Read the model definition and answer for the solid it produces. Units are mm, in the model's axes. Face numbers are marked on the shaded views. Coordinates: 2 decimals unless noted, no trailing zeros. Loops run counter-clockwise (first coordinate to the right, second up) from the corner with the lowest first, then second, coordinate; pieces in that order, holes last. Notation, with made-up numbers: M 47,54 L 95,54 A19 cw 95,73 Z; hole C 55,36.5 d8. An arc over 180 degrees is marked long. One line per item, written item: value. Start each with the question number.
1. The part is cut by section A-A (y = 53). Write down the section's boundary in (x, z), then the cut area to 3 significant figures.
2. The part is cut by section B-B (x = 76). Write down the section's boundary in (y, z), then the cut area to 3 significant figures.
3. Flat-ended cylindrical pins translate along their axes: pin 1 (4.5 mm diameter, centred on x = 32.21, y = 39.51, fed in from +Z); pin 2 (2 mm diameter, centred on y = 47.5, z = 3, fed in from -X); pin 3 (1 mm diameter, centred on x = 90.5, z = 3, fed in from +Y); pin 4 (1.1 mm diameter, centred on y = 164.5, z = 3.5, fed in from +X). Find the tip coordinate at first contact, or state that the pin passes through.
4. Consider probe 1 along Y at (x, z) = (40.5, 0.5); probe 2 along Y at (x, z) = (33.5, 1.75); probe 3 along X at (y, z) = (42, 4.5). Determine where each line is inside the solid, lowest interval first.
5. Determine the mould class of the marked faces 1 and 2 for opening direction Z: +Z half, -Z half, draft (parallel to the pull), parting line (faces both ways), or undercut.
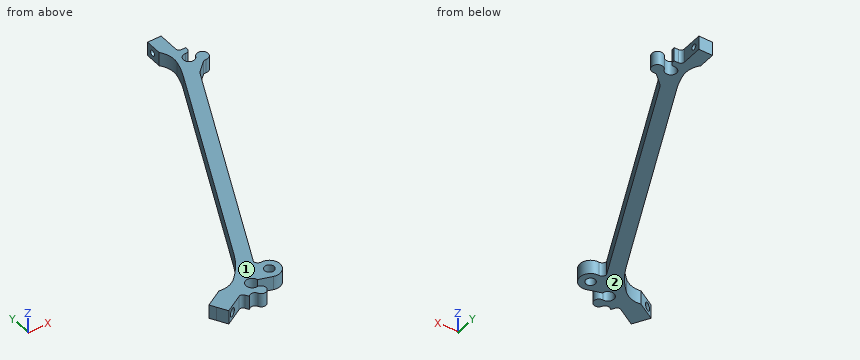
```python
from build123d import *

# Parameters (mm, degrees)
SKETCH1_R                 = 2.159
BOSS_EXTRUDE1_DEPTH       = 6.35
SKETCH2_R                 = 1.8288
CUT_EXTRUDE1_DEPTH        = 192.647335654
SKETCH3_R                 = 0.635
CUT_EXTRUDE2_DEPTH        = 192.476049021
FILLET1_R                 = 1.5875
FILLET2_R                 = 38.1
M3X0_5_TAPPED_HOLE1_D     = 2.5
M3X0_5_TAPPED_HOLE1_DEPTH = 7.50062
M3X0_5_TAPPED_HOLE1_TIP   = 0.751075774
CORTAR_EXTRUIR1_DEPTH     = 10
CROQUIS8_W                = 8.969129367
CROQUIS8_H                = 6.35
CROQUIS8_R                = 1.8288
SALIENTE_EXTRUIR3_DEPTH   = 3
CROQUIS7_W                = 6.35
CROQUIS7_H                = 7.383174339
CROQUIS7_R                = 1.25
SALIENTE_EXTRUIR4_DEPTH   = 3
REDONDEO1_R               = 10


with BuildPart() as part:
    # Sketch1 → Boss-Extrude1 (new body)
    with BuildSketch(Plane.XY):
        with BuildLine():
            Line((15.834722261, 31.434493723), (25.183466494, 36.831993723))
            Line((25.183466494, 36.831993723), (26.929716494, 33.8074))
            Line((26.929716494, 33.8074), (27.78608986, 34.301827393))
            ThreePointArc((27.78608986, 34.301827393), (29.23868298, 34.44834582), (30.311273673, 33.457869357))
            ThreePointArc((30.311273673, 33.457869357), (34.825897025, 33.143744407), (32.428977808, 36.9824))
            ThreePointArc((32.428977808, 36.9824), (30.032058591, 40.821055593), (34.546681944, 40.506930643))
            ThreePointArc((34.546681944, 40.506930643), (34.984344673, 39.889437479), (35.639187691, 39.509928464))
            Line((35.639187691, 39.509928464), (40.774282272, 37.860721969))
            ThreePointArc((40.774282272, 37.860721969), (47.368100791, 42.064756802), (42.017768622, 47.767939879))
            ThreePointArc((42.017768622, 47.767939879), (40.437125748, 48.5456558), (40.301653082, 50.302050149))
            Line((40.301653082, 50.302050149), (87.227692295, 149.642175178))
            ThreePointArc((87.227692295, 149.642175178), (87.739785188, 150.497310852), (88.408996906, 151.235993347))
            Line((88.408996906, 151.235993347), (92.404798917, 154.858512458))
            ThreePointArc((92.404798917, 154.858512458), (93.060884875, 155.23586864), (93.814481006, 155.3061491))
            ThreePointArc((93.814481006, 155.3061491), (96.343832869, 159.058865136), (91.821, 158.9024))
            ThreePointArc((91.821, 158.9024), (87.298167131, 158.745934864), (89.827518994, 162.4986509))
            ThreePointArc((89.827518994, 162.4986509), (91.22159212, 162.932303457), (91.821, 164.263545213))
            Line((91.821, 164.263545213), (91.821, 165.2524))
            Line((91.821, 165.2524), (88.3285, 165.2524))
            Line((88.3285, 165.2524), (88.3285, 176.0474))
            Line((88.3285, 176.0474), (85.1535, 176.0474))
            Line((85.1535, 176.0474), (85.1535, 160.118189826))
            Line((85.1535, 160.118189826), (31.375529243, 46.272861553))
            Line((31.375529243, 46.272861553), (13.294722261, 35.833902774))
            Line((13.294722261, 35.833902774), (15.834722261, 31.434493723))
        make_face()
        with Locations((42.327648174, 42.6974)):
            Circle(SKETCH1_R, mode=Mode.SUBTRACT)
    extrude(amount=BOSS_EXTRUDE1_DEPTH)

    # Sketch2 → Cut-Extrude1 (cut, through all)
    with BuildSketch(Plane(origin=(-9.652854494, 16.719234422, 0), x_dir=(-0.8660254037844398, -0.49999999999999806, 0), z_dir=(0.499999999999998, -0.8660254037844397, 0))):
        with Locations(Location((-32.605518601, -3.175, 0), (0, 0, 180))):
            Circle(SKETCH2_R)
    extrude(amount=-CUT_EXTRUDE1_DEPTH, mode=Mode.SUBTRACT)

    # Sketch3 → Cut-Extrude2 (cut, through all)
    with BuildSketch(Plane(origin=(88.3285, 0, 0), x_dir=(0, 0, -1), z_dir=(1, 0, 0))):
        with Locations((-3.175, 172.8724)):
            Circle(SKETCH3_R)
    extrude(amount=-CUT_EXTRUDE2_DEPTH, mode=Mode.SUBTRACT)

    # Fillet1
    fillet1_edges = [part.edges().sort_by_distance(p)[0] for p in [
        (88.3285, 165.2524, 3.175),
        (25.183466494, 36.831993723, 3.175),
    ]]
    fillet(fillet1_edges, radius=FILLET1_R)

    # Fillet2
    fillet2_edges = [part.edges().sort_by_distance(p)[0] for p in [
        (31.375529243, 46.272861553, 3.175),
        (85.1535, 160.118189826, 3.175),
    ]]
    fillet(fillet2_edges, radius=FILLET2_R)

    # M3x0.5 Tapped Hole1
    with Locations(Plane.ZY.offset(-85.1535)):
        with Locations((3.175, 172.8724)):
            Hole(M3X0_5_TAPPED_HOLE1_D / 2, depth=M3X0_5_TAPPED_HOLE1_DEPTH)
            with Locations((0, 0, -(M3X0_5_TAPPED_HOLE1_DEPTH + M3X0_5_TAPPED_HOLE1_TIP / 2))):  # 118° drill point
                Cone(0, M3X0_5_TAPPED_HOLE1_D / 2, M3X0_5_TAPPED_HOLE1_TIP, mode=Mode.SUBTRACT)

    # Croquis1 → Cortar-Extruir1 (cut)
    with BuildSketch(Plane(origin=(0, 0, 0), x_dir=(-1, 0, 0), z_dir=(0, 0, -1))):
        with BuildLine():
            ThreePointArc((-42.017768622, 47.767939879), (-47.368100791, 42.064756802), (-40.774282272, 37.860721969))
            Line((-40.774282272, 37.860721969), (-35.639187691, 39.509928464))
            ThreePointArc((-35.639187691, 39.509928464), (-34.984344673, 39.889437479), (-34.546681944, 40.506930643))
            ThreePointArc((-34.546681944, 40.506930643), (-30.032058591, 40.821055593), (-32.428977808, 36.9824))
            ThreePointArc((-32.428977808, 36.9824), (-34.825897025, 33.143744407), (-30.311273673, 33.457869357))
            ThreePointArc((-30.311273673, 33.457869357), (-29.23868298, 34.44834582), (-27.78608986, 34.301827393))
            Line((-27.78608986, 34.301827393), (-26.94132658, 33.814103086))
            ThreePointArc((-26.94132658, 33.814103086), (-28.820278114, 34.784830402), (-30.541333264, 33.555708942))
            ThreePointArc((-30.541333264, 33.555708942), (-34.611603925, 33.272501802), (-32.450601953, 36.733336963))
            ThreePointArc((-32.450601953, 36.733336963), (-29.998259186, 41.214498053), (-34.957952736, 39.991293387))
            Line((-34.957952736, 39.991293387), (-40.850727445, 38.098747463))
            ThreePointArc((-40.850727445, 38.098747463), (-47.12004702, 42.095890817), (-42.0330186, 47.518405436))
            ThreePointArc((-42.0330186, 47.518405436), (-40.565017979, 48.024188561), (-39.885018398, 49.420054945))
            Line((-39.885018398, 49.420054945), (-40.301653082, 50.302050149))
            ThreePointArc((-40.301653082, 50.302050149), (-40.437125748, 48.5456558), (-42.017768622, 47.767939879))
        make_face()
    extrude(amount=-CORTAR_EXTRUIR1_DEPTH, mode=Mode.SUBTRACT)

    # Croquis8 → Saliente-Extruir3 (add)
    with BuildSketch(Plane(origin=(-12.192854494, 21.118643474, 0), x_dir=(0.8660254037844494, 0.4999999999999815, 0), z_dir=(-0.49999999999998146, 0.8660254037844493, 0))):
        with Locations((33.915083284, -3.175)):
            Rectangle(CROQUIS8_W, CROQUIS8_H)
        with Locations((32.605518601, -3.175)):
            Circle(CROQUIS8_R, mode=Mode.SUBTRACT)
    extrude(amount=SALIENTE_EXTRUIR3_DEPTH)

    # Croquis7 → Saliente-Extruir4 (add)
    with BuildSketch(Plane.ZY.offset(-85.1535)):
        with Locations((3.175, 172.355812831)):
            Rectangle(CROQUIS7_W, CROQUIS7_H)
        with Locations((3.175, 172.8724)):
            Circle(CROQUIS7_R, mode=Mode.SUBTRACT)
    extrude(amount=SALIENTE_EXTRUIR4_DEPTH)

    # Redondeo1
    # the kernel refuses this fillet: 10 mm, written as the material it adds along each edge
    with BuildSketch(Plane(origin=(21.062216142, 40.318467458, 0), x_dir=(-0.49999999999998396, 0.8660254037844479, 0), z_dir=(0, 0, 1))) as redondeo1_piece_1:
        with BuildLine():
            CenterArc((10.726495726, -6.348327637), REDONDEO1_R, 140.592418032, 52.464514334)
            Line((0.985035131, -8.607518967), (0.790205919, -8.652702794))
            ThreePointArc((0.790205919, -8.652702794), (0.048356716, -4.354588769), (-0.2, 0))
            Line((-0.2, 0), (0, 0.2))
            ThreePointArc((0, 0.2), (1.5, 0.2), (2.845470085, 0.126966553))
            Line((2.845470085, 0.126966553), (3, 0))
        make_face()
    extrude(amount=6.35)
    with BuildSketch(Plane(origin=(85.1535, 168.664225661, 0), x_dir=(-0.1136968347067967, -0.9935154904568199, 0), z_dir=(0, 0, 1))) as redondeo1_piece_2:
        with BuildLine():
            CenterArc((7.526730458, -9.935154905), REDONDEO1_R, 83.471533817, 52.464514334)
            Line((0.341090504, -2.980546471), (0.197377705, -2.841454303))
            ThreePointArc((0.197377705, -2.841454303), (-0.028157846, -1.513012603), (-0.198703098, -0.022739367))
            Line((-0.198703098, -0.022739367), (-0.022739367, 0.198703098))
            ThreePointArc((-0.022739367, 0.198703098), (4.331849402, 0.447059814), (8.686438172, 0.198703098))
            Line((8.686438172, 0.198703098), (8.663698805, 0))
        make_face()
    extrude(amount=6.35)


solid = part.part
```
Answer block:
1. outline: M 34.24,0 L 41.58,0 L 41.58,6.35 L 34.24,6.35 Z
1. area: 46.6 mm2
2. outline: M 125.87,0 L 140.74,0 L 140.74,6.35 L 125.87,6.35 Z
2. area: 94.4 mm2
3. pin 1: passes through
3. pin 2: stops at x = 29.08
3. pin 3: stops at y = 165.25
3. pin 4: stops at x = 91.82
4. probe 1: y = 38.21 to 41.55, 43.85 to 48.08, 50.72 to 65.59
4. probe 2: y = 32.33 to 36.58, 41.99 to 51.86
4. probe 3: x = 17.97 to 30.95, 33.47 to 40.28, 44.37 to 47.11
5. face 1: +Z half
5. face 2: -Z half
